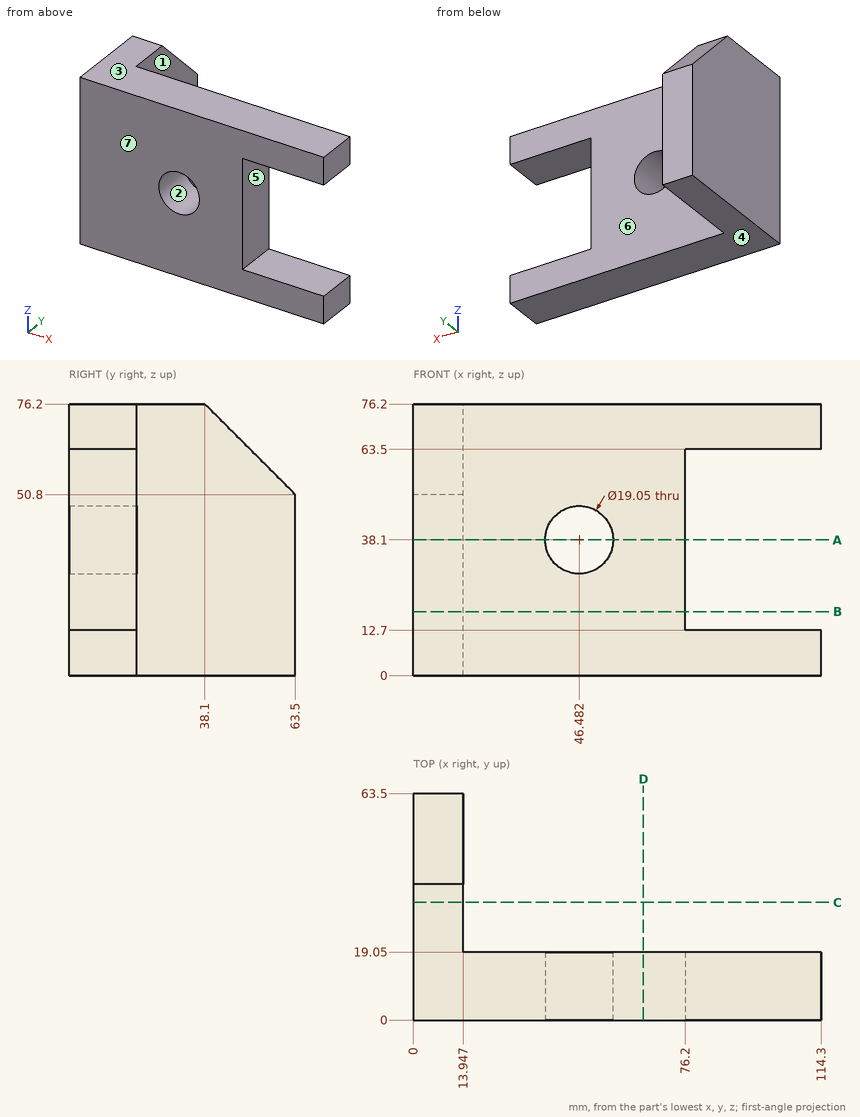
Study the drawing (mm; zero at the part's minimum x, y, z) and answer. A direction names the side the tool comes from. Give positions to 0.01 mm unless a question says otherwise; leave off trailing zeros. Order: outer loops, then holes, each group sorted by start corner. A loop starts at its lowest first (then second) coordinate and runs counter-clockwise, first axis right, second up. Notation, with made-up numbers: (34, -11) - (86, -11) arc R22 ccw to (86, 20) - close; hole circle Ø10 at (-8, -10). An arc over 180 degrees is marked (long way). Answer in a Markdown table with one row per item. Add a question column.
Q1. For a pull along Z with two mould halves and no side action, classify the marked faces 1, 2, 3 and 4 as released by +Z, released by -Z, zero draft, split by the parting line, or undercut.
Q2. The part is cut by section A-A (z = 38.1). Determine the outline of the cut face in (x, y), then the cut area to 3 significant figures.
Q3. The part is cut by section C-C (y = 33). Determine the outline of the cut face in (x, z).
Q4. Given P1, Ø21, axis at y = 13, z = 34.5, coming from the +X side; P2, Ø1.5, axis at y = 39.5, z = 49.5, coming from the +X side; P3, Ø12, axis at x = 66, z = 46, coming from the +Y side, each flat-ended and moving along its own axis, determine where each tip first touches the part or whether it passes through.
Q5. The part is cut by section D-D (x = 64.5). Determine the outline of the cut face in (y, z), then the cut area to 3 significant figures.
Q6. The part is cut by section B-B (z = 18). Determine the outline of the cut face in (x, y).
Q7. Find the intervals of material crossed by line 1 along Z through (x, y) = (46, 5); line 2 along X through (y, z) = (6, 38); line 3 along Y through (x, z) = (37.5, 44), in increasing order. Write a range as [from, to].
Q8. Which of the six approach directions +Z, -Z, +X, -X, +Y, -Y give full straight-line access (tool end or side, diameter ignored) to the marked faces 5, 6 and 7?
Determined:
| question | item | result |
|---|---|---|
| 1 | face 1 | zero draft |
| 1 | face 2 | undercut |
| 1 | face 3 | released by +Z |
| 1 | face 4 | released by -Z |
| 2 | outline | (0, 0) - (36.96, 0) - (36.96, 19.05) - (13.95, 19.05) - (13.95, 63.5) - (0, 63.5) - close; (56.01, 0) - (76.2, 0) - (76.2, 19.05) - (56.01, 19.05) - close |
| 2 | area | 1,710 mm² |
| 3 | outline | (0, 0) - (13.95, 0) - (13.95, 76.2) - (0, 76.2) - close |
| 4 | P1 | stops at x = 76.2 |
| 4 | P2 | stops at x = 13.95 |
| 4 | P3 | stops at y = 19.05 |
| 5 | outline | (0, 0) - (19.05, 0) - (19.05, 76.2) - (0, 76.2) - close |
| 5 | area | 1,450 mm² |
| 6 | outline | (0, 0) - (76.2, 0) - (76.2, 19.05) - (13.95, 19.05) - (13.95, 63.5) - (0, 63.5) - close |
| 7 | line 1 | z = [0, 28.59], [47.61, 76.2] |
| 7 | line 2 | x = [0, 36.96], [56.01, 76.2] |
| 7 | line 3 | y = [0, 19.05] |
| 8 | face 5 | +X, +Y, -Y |
| 8 | face 6 | +Z, -Z, +X, +Y |
| 8 | face 7 | +Z, -Z, +X, -X, -Y |
